Here's the drawing with two shaded views (mm, measured from the low corner). I have some questions. Coordinates: 2 decimals unless noted, no trailing zeros. Order: outer loops, then holes, each group sorted by start corner. A loop starts at its lowest first (then second) coordinate and runs counter-clockwise, first axis right, second up. Notation, with made-up numbers: (-26.5, -33) - (-10.5, -33) arc R16 cw to (-10.5, -6) - close; hole circle Ø4 at (8.25, 23). An arc over 180 degrees is marked (long way). Answer as CSV lines item,"result". Start each with the question number.
1. For pin 1 (25 mm diameter, centred on y = 488, z = 625.5, fed in from +X); pin 2 (25 mm diameter, centred on x = 632.5, y = 485, fed in from +Z); pin 3 (4 mm diameter, centred on x = 111, z = 429, fed in from -Y), each with a flat end and sliding along its axis, tell me the tip position at first contact or that it passes through.
2. I want a section at A-A, the plane y = 97. List the corners of the cut face in (x, z) for me, and give its area (3 significant figures).
3. I need wall thicknesses on probe 1 along X at (y, z) = (117.5, 599). Which ranges of the line are inside material? Lowest first, please.
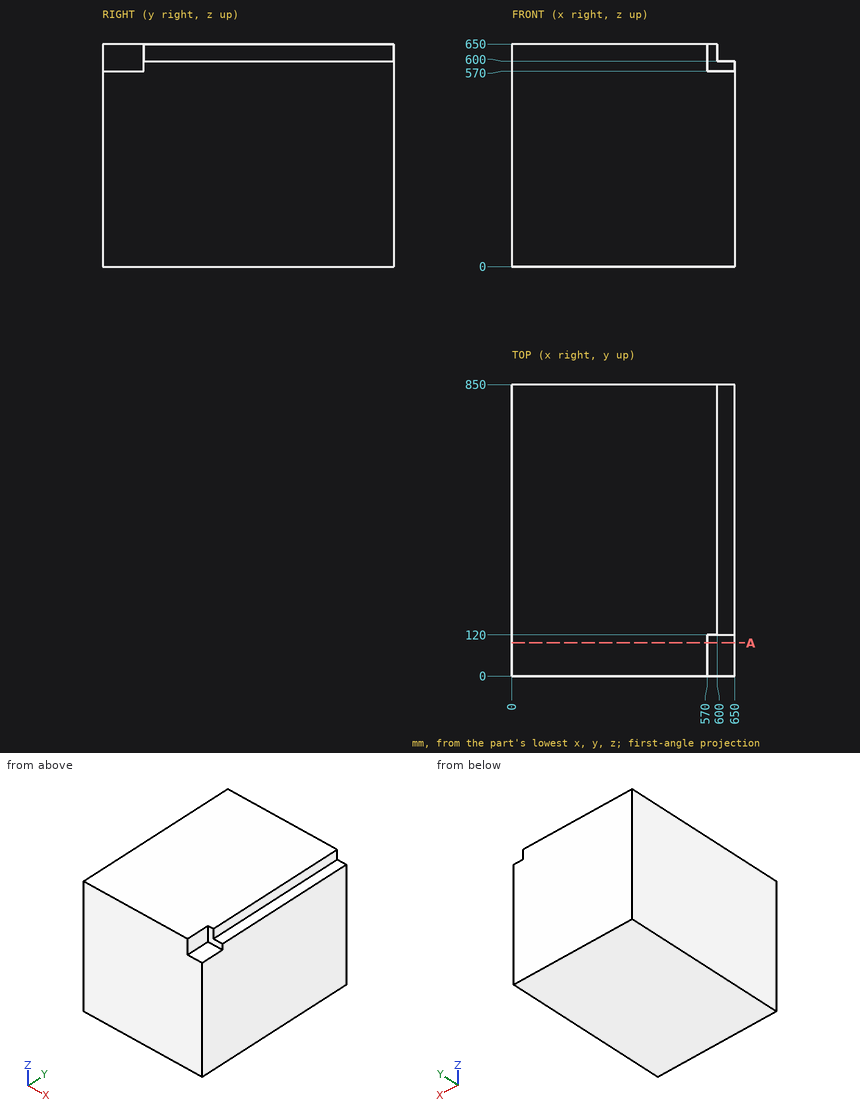
Solved:
1,pin 1,"stops at x = 600"
1,pin 2,"stops at z = 600"
1,pin 3,"stops at y = 0"
2,outline,"(0, 0) - (650, 0) - (650, 570) - (570, 570) - (570, 650) - (0, 650) - close"
2,area,"416,000 mm2"
3,probe 1,"x = 0 to 570"
